Verification items for the finished model (mm, model axes). A direction names the side the tool comes from. Coordinates: 2 decimals unless noted, no trailing zeros. Write each loop counter-clockwise with the first axis right and the second up, starting at its lowest first coordinate (ties: lowest second). Pieces come first, ordered by that corner, then holes. Notation, with made-up numbers: (-24, -6) -> (21, -6) arc R25 ccw to (21, 27) -> close; hole circle Ø7 at (17.5, -36.5). An arc over 180 degrees is marked (long way). Write item = value, one per line. Start each with the question number.
(1) Gauge pin test, flat ends, axial feed: pin 1 Ø10 at (x, z) = (-5, -3.5) entering from +Y; pin 2 Ø2 at (x, y) = (0.5, 48) entering from +Z; pin 3 Ø0.8 at (y, z) = (19, -0.5) entering from -X. Record the tip position at first contact, or that the pin passes through.
(2) Section check D-D (y = 13). Record the cut outline in (x, z), plus the area to 3 significant figures.
(3) Mould release check, pull along Z, two halves, no side actions. Record for faces 1 (the face through (0, 1.2, -5)), 2 (the face through (0, 20, -1.05)), 3 (the face through (0, 20, 0)), 4 (the face through (8.8, 11.7, -0.5)): released by +Z, released by -Z, zero draft, split by the parting line, or undercut.
(4) Section check C-C (z = -39). Record the cut outline in (x, y).
(5) Material ranges on probe 1 along Z at (x, y) = (0, 25); probe 2 along Z at (x, y) = (0, 48); probe 3 along Z at (x, y) = (-4.5, 21), recorded low to high. Write a range as [from, to].
(6) Section check B-B (x = 0). Record the cut outline in (y, z).
(7) Set-up check for faces 5 (the face through (8.8, 28.3, -0.5)), 6 (the face through (-8.8, 11.7, -0.5)), 7 (the face through (0, 40, -4)): record each of +Z, -Z, +X, -X, +Y, -Y from which the full face is reachable in a straight line by a thin tool's end or side.
(8) Section check A-A (y = 26). Record the cut outline in (x, z).
Autodesk Inventor part; units mm, degrees
ref_plane "YZ Plane" through (0, 0, 0) normal (1, 0, 0) x (0, 1, 0)
ref_plane "XZ Plane" through (0, 0, 0) normal (0, 1, 0) x (-1, 0, 0)
ref_plane "XY Plane" through (0, 0, 0) normal (0, 0, 1) x (1, 0, 0)
sketch "Szkic1" plane through (0, 0, 0) normal (0, 1, 0) x (-1, 0, 0)
  circle A0 centre (0, -30) radius 20
  line L0 (12.5, 0) -> (-12.5, 0)
  line L1 (-12.5, 0) -> (-12.5, -1.05)
  line L2 (-12.5, -1.05) -> (12.5, -1.05)
  line L3 (12.5, -1.05) -> (12.5, 0)
  circle A1 centre (0, -30) radius 21
  line L4 (-2, -9.0955) -> (2, -9.0955)
  line L5 (2, -9.0955) -> (2, -1.05)
  line L6 (2, -1.05) -> (-2, -1.05)
  line L7 (-2, -1.05) -> (-2, -9.0955)
  point P0 (0, 0)
  point P1 (0, -1.05)
  point P2 (0, 0)
  point P3 (0, -9.0955)
  dimension "d15" = 40
  dimension "d16" = 25
  dimension "d17" = 1.05
  dimension "d18" = 30
  dimension "d19" = 1
  dimension "d20" = 4
extrude "Wyciągnięcie proste1" add sketch "Szkic1" along normal blind 40 contours L3 L2 L1 L0
extrude "Extrusion2" add sketch "Szkic1" along normal blind 1.2 contours L5 A1 L7 L2 | L4 A1 picked at (0.2225, -9.0672)
sketch "Sketch2" plane through (-12.5, 0, 0) normal (0, 0, 1) x (1, 0, 0)
  line L0 (25, 40) -> (0, 40)
  line L1 (25, 0) -> (25, 40)
  line L2 (0, 40) -> (25, 40)
  line L3 (25, 40) -> (25, 32)
  line L4 (25, 32) -> (13, 20)
  line L5 (25, 8) -> (25, 0)
  line L6 (0, 0) -> (0, 40)
  line L7 (25, 0) -> (0, 0)
  line L8 (0, 0) -> (0, 8)
  line L9 (12, 20) -> (0, 32)
  line L10 (0, 32) -> (0, 40)
  line L11 (17.5, 60) -> (27.5, 60) construction
  line L12 (0, 20) -> (25, 20) construction
  line L13 (0, 8) -> (12, 20)
  line L14 (25, 8) -> (13, 20)
  line L15 (12.5, 40) -> (12.5, 0) construction
  line L16 (0, 40) -> (25, 40) construction
  line L17 (0, 0) -> (25, 0) construction
  line L18 (7.5, 15.5) -> (7.5, 24.5)
  line L19 (17.5, 15.5) -> (17.5, 24.5)
  point P0 (0, 32)
  dimension "d24" = 45
  dimension "d26" = 8
  dimension "d48" = 8
  dimension "d49" = 10
extrude "Extrusion3" cut sketch "Sketch2" against normal blind 1.2 contours L1 L14 L19 L4 | L9 L18 L13 L6
sketch "Sketch4" plane through (0, 0, 0) normal (1, 0, 0) x (0, 1, 0)
  line L0 (1.2, -9.0955) -> (1.2, -1.05)
  line L1 (38.6, -9.0955) -> (38.6, -1.05)
  line L2 (32, -1.05) -> (40, -1.05)
  line L3 (40, -1.05) -> (40, -9.0955)
  line L4 (1.2, -2.7471) -> (1.2, -1.05)
  line L5 (1.2, -1.05) -> (1.2, -9.0955)
  line L6 (32, -1.05) -> (24.5, -1.05)
  line L7 (40, -9.0955) -> (38.6, -9.0955)
  line L8 (32, -1.05) -> (40, -1.05)
  point P0 (0, 0)
  point P1 (1.2, -14.3431)
  point P2 (20, -1.05)
  point P3 (25, -1.05)
  dimension "d32" = 1.4
extrude "Extrusion4" add sketch "Sketch4" along normal mid plane 4
extrude "Extrusion5" add sketch "Szkic1" along normal blind 70 contours L4 A1 | A1 L4
extrude "Wyciągnięcie proste6" cut sketch "Szkic1" along normal blind 70 contours A0
equation "\"d26\" = d48"
equation "\"d35\" = d20"
properties part number "solo_rurka"
Response:
q1.pin_1 = 40
q1.pin_2 = -9
q1.pin_3 = -5
q2.outline = circle Ø42 at (0, -30); (-7.5, -1.05) -> (7.5, -1.05) -> (7.5, 0) -> (-7.5, 0) -> close; hole circle Ø40 at (0, -30)
q2.area = 145 mm2
q3.face_1 = undercut
q3.face_2 = undercut
q3.face_3 = released by +Z
q3.face_4 = zero draft
q4.outline = (-18.97, 0) -> (-17.86, 0) -> (-17.86, 70) -> (-18.97, 70) -> close; (17.86, 0) -> (18.97, 0) -> (18.97, 70) -> (17.86, 70) -> close
q5.probe_1 = [-51, -50], [-10, -9], [-1.05, 0]
q5.probe_2 = [-51, -50], [-10, -9]
q5.probe_3 = [-50.51, -49.49], [-10.51, -9.49], [-1.05, 0]
q6.outline = (0, -51) -> (70, -51) -> (70, -50) -> (0, -50) -> close; (0, -10) -> (70, -10) -> (70, -9) -> (40, -9) -> (40, 0) -> (0, 0) -> close; hole (1.2, -9) -> (38.6, -9) -> (38.6, -1.05) -> (1.2, -1.05) -> close
q7.face_5 = +Z, +X
q7.face_6 = +Z, -X
q7.face_7 = +Z, +X, -X, +Y
q8.outline = circle Ø42 at (0, -30); (-6.5, -1.05) -> (6.5, -1.05) -> (6.5, 0) -> (-6.5, 0) -> close; hole circle Ø40 at (0, -30)
